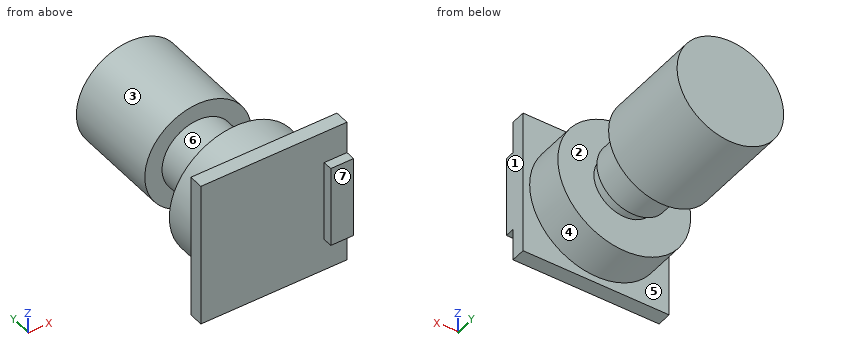
from build123d import *

# Parameters (mm, degrees)
SKETCH1_W           = 38.5
SKETCH1_H           = 38.5
BOSS_EXTRUDE1_DEPTH = 3.8
SKETCH2_R           = 17.5
BOSS_EXTRUDE2_DEPTH = 10.7
SKETCH3_R           = 8
BOSS_EXTRUDE3_DEPTH = 3.3
SKETCH4_R           = 9.5
BOSS_EXTRUDE4_DEPTH = 11
SKETCH5_R           = 14.05
BOSS_EXTRUDE5_DEPTH = 26
SKETCH7_W           = 6
SKETCH7_H           = 21.5
BOSS_EXTRUDE6_DEPTH = 2.5


with BuildPart() as part:
    # Sketch1 → Boss-Extrude1 (new body)
    with BuildSketch(Plane(origin=(0, 0, 0), x_dir=(1, 0, 0), z_dir=(0, 1, 0))):
        Rectangle(SKETCH1_W, SKETCH1_H)
    extrude(amount=BOSS_EXTRUDE1_DEPTH)

    # Sketch2 → Boss-Extrude2 (add)
    with BuildSketch(Plane(origin=(0, 3.8, 0), x_dir=(1, 0, 0), z_dir=(0, 1, 0))):
        Circle(SKETCH2_R)
    extrude(amount=BOSS_EXTRUDE2_DEPTH)

    # Sketch3 → Boss-Extrude3 (add)
    with BuildSketch(Plane(origin=(0, 14.5, 0), x_dir=(1, 0, 0), z_dir=(0, 1, 0))):
        Circle(SKETCH3_R)
    extrude(amount=BOSS_EXTRUDE3_DEPTH)

    # Sketch4 → Boss-Extrude4 (add)
    with BuildSketch(Plane(origin=(0, 17.8, 0), x_dir=(1, 0, 0), z_dir=(0, 1, 0))):
        Circle(SKETCH4_R)
    extrude(amount=BOSS_EXTRUDE4_DEPTH)

    # Sketch5 → Boss-Extrude5 (add)
    with BuildSketch(Plane(origin=(0, 28.8, 0), x_dir=(1, 0, 0), z_dir=(0, 1, 0))):
        Circle(SKETCH5_R)
    extrude(amount=BOSS_EXTRUDE5_DEPTH)

    # Sketch7 → Boss-Extrude6 (add)
    with BuildSketch(Plane.XZ):
        with Locations((16.25, 0)):
            Rectangle(SKETCH7_W, SKETCH7_H)
    extrude(amount=BOSS_EXTRUDE6_DEPTH)


solid = part.part
Design review of the part built by this model. Coordinates are the model's own, in mm. Face numbers are marked on the shaded views. A direction names the side the tool comes from. Coordinates: 2 decimals unless noted, no trailing zeros. Write each loop counter-clockwise with the first axis right and the second up, starting at its lowest first coordinate (ties: lowest second). Pieces come first, ordered by that corner, then holes. Notation, with made-up numbers: (-17, 21.5) - (4, 21.5) arc R34 ccw to (4, 60.5) - close; hole circle Ø11 at (38, 53). An arc over 180 degrees is marked (long way). One line per item, written item: value.
1) To check wall thickness, follow probe 1 along Y at (x, z) = (0, 9); probe 2 along Y at (x, z) = (3, 13); probe 3 along Y at (x, z) = (12.5, -9). State the ranges of each line that lie inside material, in increasing order.
Answer sheet:
probe 1: y = 0 to 14.5, 17.8 to 54.8
probe 2: y = 0 to 14.5, 28.8 to 54.8
probe 3: y = 0 to 14.5
2) Add section B-B (z = 11.5). State the section outline as (x, y) points.
Answer sheet:
outline: (-19.25, 0) - (19.25, 0) - (19.25, 3.8) - (13.19, 3.8) - (13.19, 14.5) - (-13.19, 14.5) - (-13.19, 3.8) - (-19.25, 3.8) - close; (-8.07, 28.8) - (8.07, 28.8) - (8.07, 54.8) - (-8.07, 54.8) - close
3) Add section C-C (x = -12). State the section outline as (y, z) points.
Answer sheet:
outline: (0, -19.25) - (3.8, -19.25) - (3.8, -12.74) - (14.5, -12.74) - (14.5, 12.74) - (3.8, 12.74) - (3.8, 19.25) - (0, 19.25) - close; (28.8, -7.31) - (54.8, -7.31) - (54.8, 7.31) - (28.8, 7.31) - close
4) Mouldability with a two-part tool opening along Y and no side actions: class the marked faces 4, 5, 6 and 7 as +Y half, -Y half, draft (parallel to the pull), parting line (faces both ways), or undercut.
Answer sheet:
face 4: draft
face 5: +Y half
face 6: undercut
face 7: -Y half
5) Add section D-D (z = 0). State the section outline as (x, y) points.
Answer sheet:
outline: (-19.25, 0) - (13.25, 0) - (13.25, -2.5) - (19.25, -2.5) - (19.25, 3.8) - (17.5, 3.8) - (17.5, 14.5) - (8, 14.5) - (8, 17.8) - (9.5, 17.8) - (9.5, 28.8) - (14.05, 28.8) - (14.05, 54.8) - (-14.05, 54.8) - (-14.05, 28.8) - (-9.5, 28.8) - (-9.5, 17.8) - (-8, 17.8) - (-8, 14.5) - (-17.5, 14.5) - (-17.5, 3.8) - (-19.25, 3.8) - close
6) Add section A-A (x = 0). State the section outline as (y, z) points.
Answer sheet:
outline: (0, -19.25) - (3.8, -19.25) - (3.8, -17.5) - (14.5, -17.5) - (14.5, -8) - (17.8, -8) - (17.8, -9.5) - (28.8, -9.5) - (28.8, -14.05) - (54.8, -14.05) - (54.8, 14.05) - (28.8, 14.05) - (28.8, 9.5) - (17.8, 9.5) - (17.8, 8) - (14.5, 8) - (14.5, 17.5) - (3.8, 17.5) - (3.8, 19.25) - (0, 19.25) - close
7) For the marked faces 1, 2 and 3, list the 3-axis set-ups (+Z, -Z, +X, -X, +Y, -Y) from which the entire face can be reached by the end or side of a thin tool; tool diameter is ignored.
Answer sheet:
face 1: +Z, -Z, +X, +Y, -Y
face 2: none
face 3: +Y
8) Insertion check: pin 1 (8 mm diameter, centred on y = 14, z = -9.5, fed in from -X); pin 2 (2 mm diameter, centred on y = -2, z = -5, fed in from -X); pin 3 (1 mm diameter, centred on y = 30, z = -4, fed in from -X). Each pin has a flat end and moves straight along its axis. Give the tip position at first contact, or say it passes through.
Answer sheet:
pin 1: stops at x = -16.61
pin 2: stops at x = 13.25
pin 3: stops at x = -13.61
